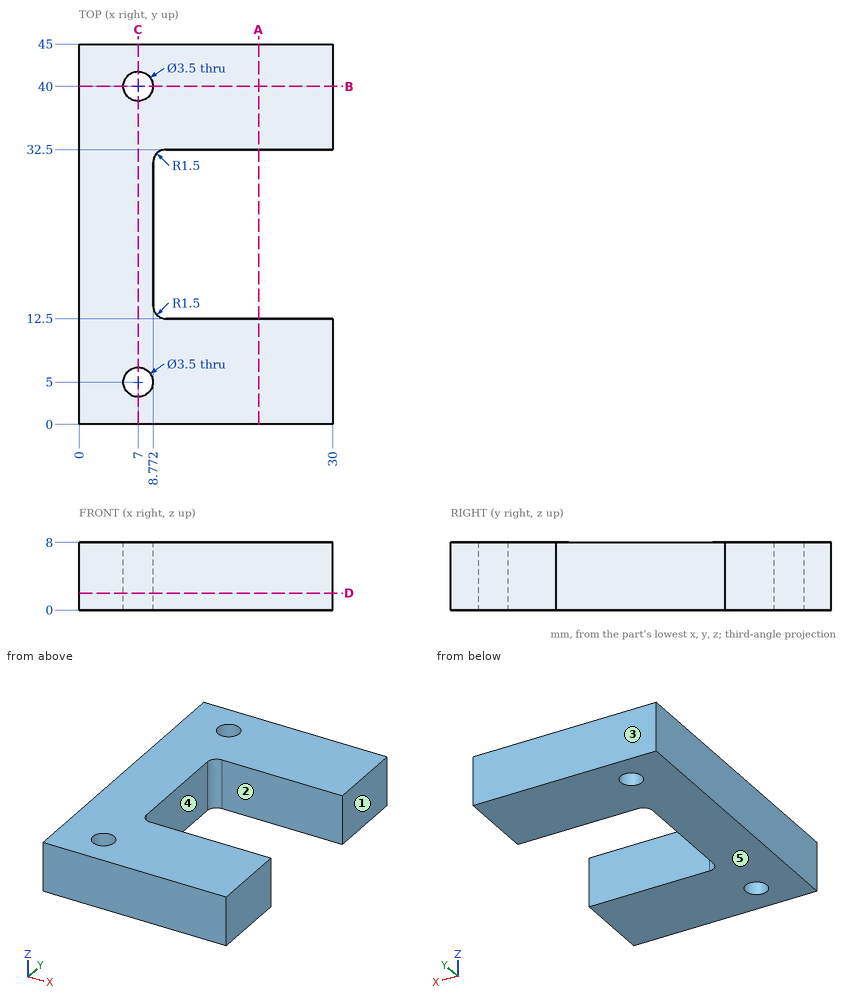
Geometry: see drawing. Coordinates: mm, zero at the bounding-box minimum. A direction names the side the tool comes from. Give positions to 0.01 mm unless a question says otherwise; leave off trailing zeros. Order: outer loops, then holes, each group sorted by start corner. A loop starts at its lowest first (then second) coordinate and runs counter-clockwise, first axis right, second up. Notation, with made-up numbers: (-30, -13) -> (26, -13) arc R17 ccw to (26, -5) -> close; hole circle Ø1 at (-15.5, 36.5). An arc over 180 degrees is marked (long way). Write each question's results on one line, items separated by ' | '. Start each with the question number.
1) First-contact query: pin 1 (2.5 mm diameter, centred on y = 22, z = 2.5, fed in from +X). Flat tip, straight axial feed; report the tip coordinate or a pass-through.
2) Section D-D (z = 2). Return loops of the section in (x, y).
3) Draft query along Y for the marked faces 3, 4 and 5. Return one class per face: pulls with the +Y half, pulls with the -Y half, needs draft (parallel to the pull), parting line crosses it, or undercut.
4) Line query: line 1 (Y direction, x = 7, z = 5.5); line 2 (Y direction, x = 20.25, z = 6.5); line 3 (Y direction, x = 6, z = 3.75). Output: solid intervals per line, ascending. Write a range as from..to.
5) Section C-C (x = 7). Return loops of the section in (y, z).
6) Section A-A (x = 21.25). Return loops of the section in (y, z), then the cut area to 3 significant figures.
7) Section B-B (y = 40). Return loops of the section in (x, z), then the cut area to 3 significant figures.
8) Set-up query: the marked faces 1 and 2. Return all of +Z, -Z, +X, -X, +Y, -Y with unobstructed straight access to the full face (end or side cutting, diameter ignored); none if empty.
Calculated:
1) pin 1: x = 8.77
2) outline: (0, 0) -> (30, 0) -> (30, 12.5) -> (10.27, 12.5) arc R1.5 cw to (8.77, 14) -> (8.77, 31) arc R1.5 cw to (10.27, 32.5) -> (30, 32.5) -> (30, 45) -> (0, 45) -> close; hole circle Ø3.5 at (7, 5); hole circle Ø3.5 at (7, 40)
3) face 3: pulls with the +Y half | face 4: undercut | face 5: needs draft
4) line 1: 0..3.25, 6.75..38.25, 41.75..45 | line 2: 0..12.5, 32.5..45 | line 3: 0..3.56, 6.44..38.56, 41.44..45
5) outline: (0, 0) -> (3.25, 0) -> (3.25, 8) -> (0, 8) -> close; (6.75, 0) -> (38.25, 0) -> (38.25, 8) -> (6.75, 8) -> close; (41.75, 0) -> (45, 0) -> (45, 8) -> (41.75, 8) -> close
6) outline: (0, 0) -> (12.5, 0) -> (12.5, 8) -> (0, 8) -> close; (32.5, 0) -> (45, 0) -> (45, 8) -> (32.5, 8) -> close | area: 200 mm2
7) outline: (0, 0) -> (5.25, 0) -> (5.25, 8) -> (0, 8) -> close; (8.75, 0) -> (30, 0) -> (30, 8) -> (8.75, 8) -> close | area: 212 mm2
8) face 1: +Z, -Z, +X, +Y, -Y | face 2: +Z, -Z, +X
